Geometry: final body of the model. Coordinates: model frame, mm. Face numbers are marked on the shaded views. Round coordinates to 2 decimals unless told otherwise and drop trailing zeros. Write each loop counter-clockwise with the first axis right and the second up, starting at its lowest first coordinate (ties: lowest second). Pieces come first, ordered by that corner, then holes. Notation, with made-up numbers: M -3.75,32 L 23.25,32 A29 ccw 23.25,63 Z; hole C 45,-2 d1. An arc over 180 degrees is marked long. Put each result on its own line as item: value. Start each with the question number.
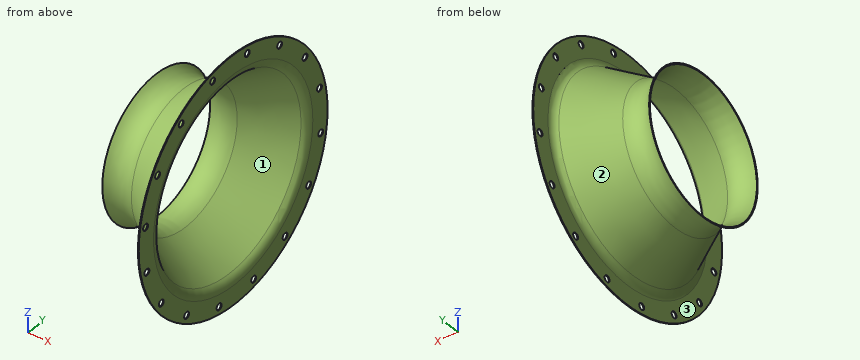
Autodesk Inventor part; units mm, degrees
ref_plane "YZ Plane" through (0, 0, 0) normal (1, 0, 0) x (0, 1, 0)
ref_plane "XZ Plane" through (0, 0, 0) normal (0, 1, 0) x (-1, 0, 0)
ref_plane "XY Plane" through (0, 0, 0) normal (0, 0, 1) x (1, 0, 0)
sketch "Sketch1" plane through (0, 0, 0) normal (0, 0, 1) x (1, 0, 0)
  line L0 (3092.83, 432.2356) -> (3090.4487, 432.2356)
  line L1 (2947.7667, 269.7223) -> (3077.9198, 348.6127)
  line L2 (2946.5323, 271.7587) -> (3076.6855, 350.6491)
  arc A0 (3077.9198, 348.6127) -> (3092.83, 375.0856) centre (3061.8737, 375.0856) ccw
  arc A1 (3076.6855, 350.6491) -> (3090.4487, 375.0856) centre (3061.8737, 375.0856) ccw
  arc A2 (2863.2209, 274.0445) -> (2947.7667, 269.7223) centre (2908.68, 334.2074) ccw
  arc A3 (2863.2209, 277.0574) -> (2946.5323, 271.7587) centre (2908.68, 334.2074) ccw
  line L3 (2863.2209, 67.1106) -> (3092.83, 67.1106) construction
  line L4 (3090.4487, 375.0856) -> (3090.4487, 432.2356)
  line L5 (2863.2209, 277.0574) -> (2863.2209, 274.0445)
  line L6 (3092.83, 432.2356) -> (3092.83, 375.0856)
  dimension "d0" = 30.9563
  dimension "d1" = 75.4062
  dimension "d2" = 30.9563
  dimension "d3" = 153.1937
  dimension "d4" = 229.6091
  dimension "d5" = 365.125
  dimension "d6" = 209.9469
  dimension "d7" = 307.975
  dimension "d8" = 267.0969
  dimension "d9" = 2.3813
revolve "Revolution1" add sketch "Sketch1" angle 360 about axis through (2863.2209, 67.1106, 0) along (1, 0, 0)
sketch "Sketch2" plane through (3092.83, 67.1106, 0) normal (1, 0, 0) x (0, 0, -1)
  circle A0 centre (0, 0) radius 307.975
  circle A1 centre (0, 0) radius 365.125
  point P0 (333.6081, 79.2847)
  dimension "d11" = 342.9
  dimension "d12" = 79.2847
hole "Hole1" at (3092.83, 146.3953, -333.6081) direction (-1, 0, 0) diameter 19.05 end through all
pattern_circular "Circular Pattern1" count 16 over 360 about axis through (3091.6393, 67.1106, 0) along (1, 0, 0) of "Hole1"
properties part number "inlet cone" material "Steel, Mild"
1) Draft query along Y for the marked faces 1, 2 and 3. Return one class per face: +Y half, -Y half, draft (parallel to the pull), parting line (faces both ways), or undercut.
2) Section C-C, the plane x = 2936. Output: boundary loops of the cut face in (y, z).
3) Section A-A, the plane z = 0. Output: boundary loops of the cut face in (x, y).
4) First-contact query: pin 1 (22 mm diameter, centred on y = 146.4, z = -333.61, fed in from -X); pin 2 (12 mm diameter, centred on x = 3047, y = -41.5, fed in from -Z); pin 3 (17 mm diameter, centred on y = 359.07, z = -179.83, fed in from +X); pin 4 (12 mm diameter, centred on x = 2908.5, z = -4.5, fed in from -Y). Flat tips, straight axial feed; report the tip coordinate or a pass-through.
5) Section B-B, the plane x = 3030. Output: boundary loops of the cut face in (y, z).
6) Ray query, probe 1 along Z at (x, y) = (3059, 105); probe 2 along Y at (x, z) = (2990, -14); probe 3 along Y at (x, z) = (3081.5, 40). Return the intervals inside material, ascending.
Solved:
1. face 1: undercut
1. face 2: parting line
1. face 3: draft
2. outline: C 67.11,0 d398.75; hole C 67.11,0 d393.63
3. outline: M 2863.22,-142.84 A73.02 cw 2946.53,-137.54 L 3076.69,-216.43 A28.57 cw 3090.45,-240.86 L 3090.45,-298.01 L 3092.83,-298.01 L 3092.83,-240.86 A30.96 ccw 3077.92,-214.39 L 2947.77,-135.5 A75.41 ccw 2863.22,-139.82 Z; M 2863.22,274.04 A75.41 ccw 2947.77,269.72 L 3077.92,348.61 A30.96 ccw 3092.83,375.09 L 3092.83,432.24 L 3090.45,432.24 L 3090.45,375.09 A28.57 cw 3076.69,350.65 L 2946.53,271.76 A73.02 cw 2863.22,277.06 Z
4. pin 1: stops at x = 3090.45
4. pin 2: stops at z = -247.08
4. pin 3: passes through
4. pin 4: stops at y = -127.18
5. outline: C 67.11,0 d510.48; hole C 67.11,0 d504.91
6. probe 1: z = -270.17 to -267.36, 267.36 to 270.17
6. probe 2: y = -163.46 to -160.67, 294.89 to 297.68
6. probe 3: y = -217.3 to -214.09, 348.32 to 351.52
